```python
from build123d import *

# Parameters (mm, degrees)
BLANKSKE_W          = 56.5
BLANKSKE_H          = 6
BLANK_DEPTH         = 6.5
TOOTHCUTILL_DEPTH   = 58.188285514
TOOTHCUTSIM_DEPTH   = 58.188285514
TEETHCUTS_COUNT     = 13
TEETHCUTS_PITCH     = 4.712388975
SKETCH_4_W          = 19.255
SKETCH_4_H          = 6.5
SKETCH_4_W_2        = 26.245
EXTRUDE_1_DEPTH     = 2.625
SKETCH_5_W          = 16
SKETCH_5_H          = 6.5
EXTRUDE_2_DEPTH     = 3.375
SKETCH_8_R          = 1.425
CUT_EXTRUDE_1_DEPTH = 84.216494909
SKETCH_11_R         = 2.425
SKETCH_11_R_2       = 1.425
CUT_EXTRUDE_2_DEPTH = 2
CUT_EXTRUDE_START   = -0.1
SKETCH_14_W         = 102
SKETCH_14_H         = 6.5
SKETCH_14_R         = 1.425
CUT_EXTRUDE_3_DEPTH = 0.1


with BuildPart() as part:
    # BlankSke → Blank (new body)
    with BuildSketch(Plane.XY):
        with Locations((28.25, 3)):
            Rectangle(BLANKSKE_W, BLANKSKE_H)
    extrude(amount=-BLANK_DEPTH)

    # TooCutSkeIll → ToothCutIll (cut, through all)
    with BuildSketch(Plane.XY):
        with BuildLine():
            Line((-1.86868349, 5.960521209), (-0.744699446, 2.872400426))
            ThreePointArc((-0.744699446, 2.872400426), (-0.60703976, 2.692998831), (-0.39137502, 2.625))
            Line((-0.39137502, 2.625), (0.39137502, 2.625))
            ThreePointArc((0.39137502, 2.625), (0.60703976, 2.692998831), (0.744699446, 2.872400426))
            Line((0.744699446, 2.872400426), (1.86868349, 5.960521209))
            ThreePointArc((1.86868349, 5.960521209), (1.890650461, 5.989149123), (1.925065047, 6))
            Line((1.925065047, 6), (1.925065047, 6.0254))
            Line((1.925065047, 6.0254), (-1.925065047, 6.0254))
            Line((-1.925065047, 6.0254), (-1.925065047, 6))
            ThreePointArc((-1.925065047, 6), (-1.890650461, 5.989149123), (-1.86868349, 5.960521209))
        make_face()
    toothcutill = extrude(amount=-TOOTHCUTILL_DEPTH, mode=Mode.SUBTRACT)

    # TooCutSkeSim → ToothCutSim (cut, through all)
    with BuildSketch(Plane.XY):
        Polygon((0.654653055, 2.625), (-0.654653055, 2.625), (-1.892297439, 6.0254), (1.892297439, 6.0254), align=None)
    toothcutsim = extrude(amount=-TOOTHCUTSIM_DEPTH, mode=Mode.SUBTRACT)

    # TeethCuts: ToothCutIll, ToothCutSim ×13
    with Locations(*[(i * TEETHCUTS_PITCH, 0, 0) for i in range(1, TEETHCUTS_COUNT)]):
        add(toothcutill, mode=Mode.SUBTRACT)
        add(toothcutsim, mode=Mode.SUBTRACT)

    # 草图4 → 凸台-拉伸1 (add)
    with BuildSketch(Plane(origin=(0, 0, 0), x_dir=(-1, 0, 0), z_dir=(0, -1, 0))):
        with Locations((9.6275, 3.25)):
            Rectangle(SKETCH_4_W, SKETCH_4_H)
        with Locations((-69.6225, 3.25)):
            Rectangle(SKETCH_4_W_2, SKETCH_4_H)
    extrude(amount=-EXTRUDE_1_DEPTH)

    # 草图5 → 凸台-拉伸2 (add)
    with BuildSketch(Plane(origin=(0, 2.625, 0), x_dir=(1, 0, 0), z_dir=(0, 1, 0))):
        with Locations((-11.255, 3.25)):
            Rectangle(SKETCH_5_W, SKETCH_5_H)
        with Locations((74.745, 3.25)):
            Rectangle(SKETCH_5_W, SKETCH_5_H)
    extrude(amount=EXTRUDE_2_DEPTH)

    # 草图8 → 切除-拉伸1 (cut, through all)
    with BuildSketch(Plane(origin=(0, 6, 0), x_dir=(1, 0, 0), z_dir=(0, 1, 0))):
        with Locations(Location((-15.255, 3.25, 0), (0, 0, 270))):
            Circle(SKETCH_8_R)
        with Locations(Location((-7.255, 3.25, 0), (0, 0, 270))):
            Circle(SKETCH_8_R)
        with Locations(Location((78.745, 3.25, 0), (0, 0, 270))):
            Circle(SKETCH_8_R)
        with Locations(Location((70.745, 3.25, 0), (0, 0, 270))):
            Circle(SKETCH_8_R)
    extrude(amount=-CUT_EXTRUDE_1_DEPTH, mode=Mode.SUBTRACT)

    # 草图11 → 切除-拉伸2 (cut)
    # profile 1 of 4: a face of its own
    with BuildSketch(Plane(origin=(0, 6, 0), x_dir=(1, 0, 0), z_dir=(0, 1, 0))):
        with Locations(Location((70.745, 3.25, 0), (0, 0, 270))):
            Circle(SKETCH_11_R)
        with Locations(Location((70.745, 3.25, 0), (0, 0, 270))):
            Circle(SKETCH_11_R_2, mode=Mode.SUBTRACT)
    # profile 2 of 4: a face of its own
    with BuildSketch(Plane(origin=(0, 6, 0), x_dir=(1, 0, 0), z_dir=(0, 1, 0))):
        with Locations(Location((78.745, 3.25, 0), (0, 0, 270))):
            Circle(SKETCH_11_R)
        with Locations(Location((78.745, 3.25, 0), (0, 0, 270))):
            Circle(SKETCH_11_R_2, mode=Mode.SUBTRACT)
    # profile 3 of 4: a face of its own
    with BuildSketch(Plane(origin=(0, 6, 0), x_dir=(1, 0, 0), z_dir=(0, 1, 0))):
        with Locations(Location((-7.255, 3.25, 0), (0, 0, 270))):
            Circle(SKETCH_11_R)
        with Locations(Location((-7.255, 3.25, 0), (0, 0, 270))):
            Circle(SKETCH_11_R_2, mode=Mode.SUBTRACT)
    # profile 4 of 4: a face of its own
    with BuildSketch(Plane(origin=(0, 6, 0), x_dir=(1, 0, 0), z_dir=(0, 1, 0))):
        with Locations(Location((-15.255, 3.25, 0), (0, 0, 270))):
            Circle(SKETCH_11_R)
        with Locations(Location((-15.255, 3.25, 0), (0, 0, 270))):
            Circle(SKETCH_11_R_2, mode=Mode.SUBTRACT)
    extrude(amount=-CUT_EXTRUDE_2_DEPTH, mode=Mode.SUBTRACT)

    # 草图14 → 切除-拉伸3 (cut)
    with BuildSketch(Plane(origin=(0, 0, 0), x_dir=(-1, 0, 0), z_dir=(0, -1, 0)).offset(CUT_EXTRUDE_START)):
        with Locations((-31.745, 3.25)):
            Rectangle(SKETCH_14_W, SKETCH_14_H)
        with Locations(Location((15.255, 3.25, 0), (0, 0, 270))):
            Circle(SKETCH_14_R, mode=Mode.SUBTRACT)
        with Locations(Location((7.255, 3.25, 0), (0, 0, 270))):
            Circle(SKETCH_14_R, mode=Mode.SUBTRACT)
        with Locations(Location((-70.745, 3.25, 0), (0, 0, 270))):
            Circle(SKETCH_14_R, mode=Mode.SUBTRACT)
        with Locations(Location((-78.745, 3.25, 0), (0, 0, 270))):
            Circle(SKETCH_14_R, mode=Mode.SUBTRACT)
    extrude(amount=CUT_EXTRUDE_3_DEPTH, mode=Mode.SUBTRACT)


solid = part.part
```
The listing builds one solid part. Answer for the finished solid, in the listing's coordinates (mm). A direction names the side the tool comes from. Coordinates: 2 decimals unless noted, no trailing zeros. Write each loop counter-clockwise with the first axis right and the second up, starting at its lowest first coordinate (ties: lowest second). Pieces come first, ordered by that corner, then holes.
Q1. Section A-A, the plane y = 1.35 is taken. Write down the section's boundary in (x, z) (3 decimals), then the cut area to 3 significant figures.
Returned:
outline: (-19.255, -6.5) - (82.745, -6.5) - (82.745, 0) - (-19.255, 0) - close; hole circle Ø2.85 at (-15.255, -3.25); hole circle Ø2.85 at (-7.255, -3.25); hole circle Ø2.85 at (70.745, -3.25); hole circle Ø2.85 at (78.745, -3.25)
area: 637 mm2
Q2. Given P1, Ø0.7, axis at x = 52, z = -4.5, coming from the +Y side (3 decimals); P2, Ø2.5, axis at x = 78.745, z = -3.25, coming from the +Y side, each flat-ended and moving along its own axis, determine where each tip first touches the part or whether it passes through.
Returned:
P1: stops at y = 2.625
P2: passes through
Q3. Section B-B, the plane z = -3.25 is taken. Give the number of separate pieces and of enclosed holes in the cut face, then the cut area to 3 significant figures.
Returned:
separate pieces: 5
enclosed holes: 0
area: 370 mm2
Q4. The mould has two halves that part along Z. Classify faces 1 (the flat face through (31, 2, 0)), 2 (the flat face through (70.78, 4, -1.67)), 3 (the flat face through (-1, 2.625, -3)): released by +Z, released by -Z, zero draft, split by the parting line, or undercut.
Returned:
face 1: released by +Z
face 2: undercut
face 3: zero draft
Q5. Find the intervals of material crossed by line 1 along X through (y, z) = (1.55, -3.25) (3 decimals); line 2 along Y through (x, z) = (71, -1.25); line 3 along Z through (x, y) = (78, 1.1), in increasing order.
Returned:
line 1: x = -19.255 to -16.68, -13.83 to -8.68, -5.83 to 69.32, 72.17 to 77.32, 80.17 to 82.745
line 2: y = 0.1 to 4
line 3: z = -6.5 to -4.46, -2.04 to 0
Q6. Which of the six approach directions +Z, -Z, +X, -X, +Y, -Y give full straight-line access (tool end or side, diameter ignored) to faces 4 (the flat face through (-3.255, 4, -3)), 5 (the cylindrical face through (-6.527, 5.014, -0.937)), 6 (the cylindrical face through (-16.646, 2.077, -3.559))?
Returned:
face 4: +Z, -Z, +Y
face 5: +Y
face 6: +Y, -Y
Q7. Section C-C, the plane x = 62 is taken. Write down the section's boundary in (y, z) (3 decimals), then the cut area to 3 significant figures.
Returned:
outline: (0.1, -6.5) - (2.625, -6.5) - (2.625, 0) - (0.1, 0) - close
area: 16.4 mm2
